The listing builds one solid part. Answer for the finished solid, in the listing's coordinates (mm). Face numbers are marked on the shaded views. Give positions to 0.01 mm unless a question says otherwise; leave off trailing zeros. Loops run counter-clockwise (first coordinate to the right, second up) from the corner with the lowest first, then second, coordinate; pieces in that order, holes last. Notation, with made-up numbers: (1.25, -20) - (25.25, -20) arc R30 ccw to (25.25, 9) - close; hole circle Ø10 at (-7.75, 15.25). An arc over 180 degrees is marked (long way). Answer in a Markdown table with one row per item. Add a question column.
Autodesk Inventor part; units mm, degrees
ref_plane "YZ Plane" through (0, 0, 0) normal (1, 0, 0) x (0, 1, 0)
ref_plane "XZ Plane" through (0, 0, 0) normal (0, 1, 0) x (-1, 0, 0)
ref_plane "XY Plane" through (0, 0, 0) normal (0, 0, 1) x (1, 0, 0)
sketch "Sketch1" plane through (0, 0, 0) normal (0, 1, 0) x (-1, 0, 0)
  line L0 (0, 0) -> (160, 0)
  line L1 (160, 0) -> (160, -75)
  line L2 (160, -75) -> (0, -75)
  line L3 (0, -75) -> (0, 0)
  dimension "d0" = 160
  dimension "d1" = 75
extrude "Extrusion1" add sketch "Sketch1" along normal blind 50.8
sketch "Sketch2" plane through (0, 50.8, 0) normal (0, 1, 0) x (1, 0, 0)
  circle A0 centre (-110, 65) radius 6.5
  line L0 (0, 75) -> (-160, 75)
  line L1 (-160, 75) -> (-160, 0)
  circle A1 centre (-90, 65) radius 6.5
  circle A2 centre (-70, 65) radius 6.5
  circle A3 centre (-50, 65) radius 6.5
  point P0 (0, 0)
  dimension "d4" = 13
  dimension "d5" = 10
  dimension "d6" = 50
  dimension "d12" = 20
extrude "Extrusion2" cut sketch "Sketch2" against normal blind 50.8
sketch "Sketch3" plane through (0, 50.8, 0) normal (0, 1, 0) x (1, 0, 0)
  line L0 (0, 75) -> (-160, 75)
  line L1 (-112.5, 75) -> (-107.5, 75)
  line L2 (-107.5, 75) -> (-107.5, 70)
  line L3 (-107.5, 70) -> (-112.5, 70)
  line L4 (-112.5, 70) -> (-112.5, 75)
  circle A0 centre (-110, 65) radius 6.5
  line L5 (-87.5, 75) -> (-87.5, 70)
  line L6 (-87.5, 70) -> (-92.5, 70)
  line L7 (-92.5, 70) -> (-92.5, 75)
  line L8 (-92.5, 75) -> (-87.5, 75)
  line L9 (-67.5, 75) -> (-67.5, 70)
  line L10 (-67.5, 70) -> (-72.5, 70)
  line L11 (-72.5, 70) -> (-72.5, 75)
  line L12 (-72.5, 75) -> (-67.5, 75)
  line L13 (-47.5, 75) -> (-47.5, 70)
  line L14 (-47.5, 70) -> (-52.5, 70)
  line L15 (-52.5, 70) -> (-52.5, 75)
  line L16 (-52.5, 75) -> (-47.5, 75)
  point P0 (0, 0)
  dimension "d16" = 5
  dimension "d17" = 5
  dimension "d18" = 2.5
  dimension "d24" = 20
extrude "Extrusion3" cut sketch "Sketch3" against normal blind 50.8 contours L13 L14 L15 L0 | L2 A0 L4 L0 | L5 L6 L7 L0 | L9 L10 L11 L0 | L2 L3 L4 A0 picked at (-110, 70.5)
properties part number "Lateral"
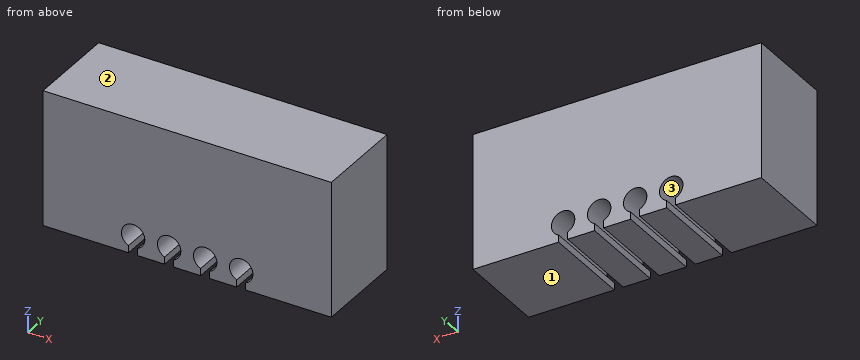
(1) A cutting plane is placed at C-C on x = -70. Determine the outline of the cut face in (y, z).
(2) A cutting plane is placed at B-B on y = 6. Determine the outline of the cut face in (x, z).
(3) A cutting plane is placed at A-A on z = -65. Determine the outline of the cut face in (x, y).
(4) The mould has two halves that part along Z. Classify the marked faces 1, 2 and 3: pulls with the +Z half, pulls with the -Z half, needs draft (parallel to the pull), parting line crosses it, or undercut.
(5) Find the intervals of material crossed by line 1 along X through (y, z) = (25, -65); line 2 along Z through (x, y) = (-90, 39); line 3 along Z through (x, y) = (-47, 15), in increasing order. Write a range as [from, to].
Evaluation:
| question | item | result |
|---|---|---|
| 1 | outline | (0, -58.5) - (50.8, -58.5) - (50.8, 0) - (0, 0) - close |
| 2 | outline | (-160, -75) - (-112.5, -75) - (-112.5, -71) arc R6.5 cw (long way) to (-107.5, -71) - (-107.5, -75) - (-92.5, -75) - (-92.5, -71) arc R6.5 cw (long way) to (-87.5, -71) - (-87.5, -75) - (-72.5, -75) - (-72.5, -71) arc R6.5 cw (long way) to (-67.5, -71) - (-67.5, -75) - (-52.5, -75) - (-52.5, -71) arc R6.5 cw (long way) to (-47.5, -71) - (-47.5, -75) - (0, -75) - (0, 0) - (-160, 0) - close |
| 3 | outline | (-160, 0) - (-116.5, 0) - (-116.5, 50.8) - (-160, 50.8) - close; (-103.5, 0) - (-96.5, 0) - (-96.5, 50.8) - (-103.5, 50.8) - close; (-83.5, 0) - (-76.5, 0) - (-76.5, 50.8) - (-83.5, 50.8) - close; (-63.5, 0) - (-56.5, 0) - (-56.5, 50.8) - (-63.5, 50.8) - close; (-43.5, 0) - (0, 0) - (0, 50.8) - (-43.5, 50.8) - close |
| 4 | face 1 | pulls with the -Z half |
| 4 | face 2 | pulls with the +Z half |
| 4 | face 3 | undercut |
| 5 | line 1 | x = [-160, -116.5], [-103.5, -96.5], [-83.5, -76.5], [-63.5, -56.5], [-43.5, 0] |
| 5 | line 2 | z = [-58.5, 0] |
| 5 | line 3 | z = [-75, -70.77], [-59.23, 0] |
